Read the model definition and answer for the solid it produces. Units are mm, in the model's axes. Face numbers are marked on the shaded views. A direction names the side the tool comes from. Give positions to 0.01 mm unless a question says otherwise; leave off trailing zeros. Loops run counter-clockwise (first coordinate to the right, second up) from the corner with the lowest first, then second, coordinate; pieces in that order, holes last. Notation, with made-up numbers: (49.5, -8.5) - (54.5, -8.5) arc R23 ccw to (54.5, 9.5) - close; hole circle Ø4 at (84, -31.75). An arc over 180 degrees is marked (long way). Use a Markdown table: item, result. Add a question column.
Item 1: A cutting plane is placed at C-C (z = 6.75). Determine the outline of the cut face in (x, y).
Item 2: Consider probe 1 along Y at (x, z) = (-6, 5.25); probe 2 along Z at (x, y) = (-3, 16.5); probe 3 along Y at (x, z) = (-3, 4.5). Determine where each line is inside the solid, lowest interval first. Write a range as [from, to].
Item 3: Each of these flat-tipped pins is pushed along its axis until it touches: P1, Ø1, axis at x = 9.5, y = -0.5, coming from the -Z side; P2, Ø16, axis at x = 10.5, y = 15, coming from the +Z side; P3, Ø4, axis at x = 4, y = -8.5, coming from the +Z side; P4, Ø3, axis at x = -1, z = 7, coming from the -Y side. Where does it stop, or does it pass through?
Item 4: A cutting plane is placed at A-A (z = 3.75). Determine the outline of the cut face in (x, y).
Item 5: Which of the six approach directions +Z, -Z, +X, -X, +Y, -Y give full straight-line access (tool end or side, diameter ignored) to the marked faces 4 and 5?
Item 6: For a pull along X with two mould halves and no side action, classify the marked faces 1, 2 and 3 as +X half, -X half, draft (parallel to the pull), parting line (faces both ways), or undercut.
Item 7: A cutting plane is placed at B-B (y = 15). Determine the outline of the cut face in (x, z).
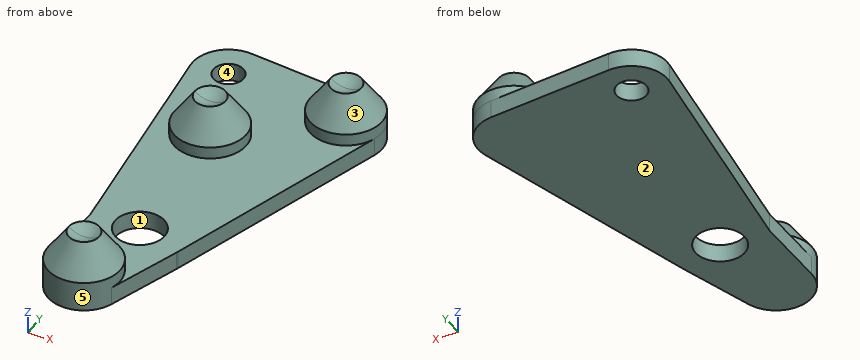
from build123d import *
from build123d.topology import SkipClean

# Parameters (mm, degrees)
BOSS_EXTRUDE1_DEPTH = 3
BOSS_EXTRUDE5_DEPTH = 3
BOSS_EXTRUDE2_DEPTH = 3
SKETCH3_R           = 4.1
CUT_EXTRUDE1_DEPTH  = 50
SKETCH1_4_R         = 6
BOSS_EXTRUDE3_DEPTH = 10
SKETCH2_4_R         = 6
BOSS_EXTRUDE4_DEPTH = 10
CHAMFER1_SIZE       = 5
CHAMFER1_SIZE_2     = 3.501037691
SKETCH9_R           = 2.5
CUT_EXTRUDE2_DEPTH  = 3


with BuildPart() as part:
    # Sketch1 → Boss-Extrude1 (new body)
    with BuildSketch(Plane.XY):
        with BuildLine():
            ThreePointArc((-7.862783113, 28.36246747), (-9.674812704, 26.016588816), (-10.142674299, 23.089524856))
            Line((-10.142674299, 23.089524856), (-7.966824047, -0.727814955))
            ThreePointArc((-7.966824047, -0.727814955), (-0.830270862, -7.956798998), (7.644946217, -2.356861757))
            Line((7.644946217, -2.356861757), (19.414515396, 35.820058514))
            ThreePointArc((19.414515396, 35.820058514), (17.084366379, 42.528936958), (9.985578884, 42.314786229))
            Line((9.985578884, 42.314786229), (-7.862783113, 28.36246747))
        make_face()
    extrude(amount=BOSS_EXTRUDE1_DEPTH)

    # Sketch8 → Boss-Extrude5 (add)
    with BuildSketch(Plane.XY):
        with BuildLine():
            Line((14.20374019, 43.56487302), (-6.42299265, 45.369478309))
            ThreePointArc((-6.42299265, 45.369478309), (-11.266837417, 43.555209842), (-12.899477398, 38.647166557))
            Line((-12.899477398, 38.647166557), (-7.938067055, -0.993524752))
            ThreePointArc((-7.938067055, -0.993524752), (-7.953555222, -0.86078995), (-7.966824047, -0.727814955))
            Line((-7.966824047, -0.727814955), (-10.142674299, 23.089524856))
            ThreePointArc((-10.142674299, 23.089524856), (-9.674812704, 26.016588816), (-7.862783113, 28.36246747))
            Line((-7.862783113, 28.36246747), (9.985578884, 42.314786229))
            ThreePointArc((9.985578884, 42.314786229), (11.97594826, 43.340396462), (14.20374019, 43.56487302))
        make_face()
    extrude(amount=BOSS_EXTRUDE5_DEPTH)

    # Sketch2 → Boss-Extrude2 (add)
    with BuildSketch(Plane.XY):
        with BuildLine():
            Line((-7.9983883, 0.16057583), (-8.256217535, -12.682068917))
            ThreePointArc((-8.256217535, -12.682068917), (-3.299315376, -18.711347307), (3.420783665, -14.741039282))
            Line((3.420783665, -14.741039282), (7.570946632, -2.584717991))
            ThreePointArc((7.570946632, -2.584717991), (-1.389185421, -7.878462024), (-7.9983883, 0.16057583))
        make_face()
    extrude(amount=BOSS_EXTRUDE2_DEPTH)

    # Sketch3 → Cut-Extrude1 (cut)
    with BuildSketch(Plane.XY.offset(3)):
        Circle(SKETCH3_R)
    extrude(amount=-CUT_EXTRUDE1_DEPTH, mode=Mode.SUBTRACT)

    # Sketch1<4> → Boss-Extrude3 (add)
    with BuildSketch(Plane.XY):
        with Locations(Location((13.680805733, 37.587704831, 0), (0, 0, 85))):
            Circle(SKETCH1_4_R)
        with Locations((-2.167556264, 25.198814555)):
            Circle(SKETCH1_4_R)
    extrude(amount=BOSS_EXTRUDE3_DEPTH)

    # Sketch2<4> → Boss-Extrude4 (add)
    with BuildSketch(Plane.XY):
        with Locations(Location((-2.25742631, -12.802500789, 0), (0, 0, 178.849883098))):
            Circle(SKETCH2_4_R)
    extrude(amount=BOSS_EXTRUDE4_DEPTH)

    # Sketch5 one side → Cut-Revolve1 (revolve, cut)
    with SkipClean():  # the faces are left unmerged after this step: merging them gives an invalid solid
        with BuildSketch(Plane(origin=(13.680805733, 0, 0), x_dir=(0, 0, -1), z_dir=(1, 0, 0))):
            with BuildLine():
                ThreePointArc((-13, 33.587704831), (-10.171572875, 34.759277707), (-9, 37.587704831))
                ThreePointArc((-9, 37.587704831), (-10.171572875, 40.416131956), (-13, 41.587704831))
                Line((-13, 41.587704831), (-13, 33.587704831))
            make_face()
        revolve(axis=Axis((13.680805733, 41.587704831, 13), (0, -1, 0)), mode=Mode.SUBTRACT)

    # Sketch6 → Cut-Revolve2 (revolve, cut)
    with SkipClean():  # the faces are left unmerged after this step: merging them gives an invalid solid
        with BuildSketch(Plane(origin=(-2.167556264, 0, 0), x_dir=(0, 0, -1), z_dir=(1, 0, 0))):
            with BuildLine():
                ThreePointArc((-9, 25.198814555), (-10.171572875, 28.02724168), (-13, 29.198814555))
                Line((-13, 29.198814555), (-13, 21.198814555))
                ThreePointArc((-13, 21.198814555), (-10.171572875, 22.37038743), (-9, 25.198814555))
            make_face()
            with BuildLine():
                Line((-13, 21.198814555), (-13, 29.198814555))
                ThreePointArc((-13, 29.198814555), (-17, 25.198814555), (-13, 21.198814555))
            make_face()
        revolve(axis=Axis((-2.167556264, 29.198814555, 13), (0, -1, 0)), mode=Mode.SUBTRACT)

    # Sketch7 → Cut-Revolve3 (revolve, cut)
    with SkipClean():  # the faces are left unmerged after this step: merging them gives an invalid solid
        with BuildSketch(Plane(origin=(-2.25742631, 0, 0), x_dir=(0, 0, -1), z_dir=(1, 0, 0))):
            with BuildLine():
                ThreePointArc((-9, -12.802500789), (-10.171572875, -9.974073664), (-13, -8.802500789))
                Line((-13, -8.802500789), (-13, -16.802500789))
                ThreePointArc((-13, -16.802500789), (-10.171572875, -15.630927914), (-9, -12.802500789))
            make_face()
            with BuildLine():
                Line((-13, -16.802500789), (-13, -8.802500789))
                ThreePointArc((-13, -8.802500789), (-17, -12.802500789), (-13, -16.802500789))
            make_face()
        revolve(axis=Axis((-2.25742631, -8.802500789, 13), (0, -1, 0)), mode=Mode.SUBTRACT)

    # Chamfer1
    # the kernel refuses this chamfer: 5, 3.501037691 mm, written as the material it takes off along each edge
    with BuildSketch(Plane(origin=(-2.25742631, -12.802500789, 10), x_dir=(-0.9997985375420249, 0.020071978697384193, 0), z_dir=(0.020071978697384193, 0.9997985375420249, 0))) as chamfer1_piece_1:
        Polygon((6, -CHAMFER1_SIZE), (6 - CHAMFER1_SIZE_2, 0), (6, 0), align=None)
    revolve(axis=Axis((-2.25742631, -12.802500789, 10), (0, 0, 1)), mode=Mode.SUBTRACT)
    with BuildSketch(Plane(origin=(13.680805733, 37.587704831, 10), x_dir=(0.08715574274765815, 0.9961946980917454, 0), z_dir=(0.9961946980917454, -0.08715574274765815, 0))) as chamfer1_piece_2:
        Polygon((6, -CHAMFER1_SIZE), (6 - CHAMFER1_SIZE_2, 0), (6, 0), align=None)
    revolve(axis=Axis((13.680805733, 37.587704831, 10), (0, 0, 1)), mode=Mode.SUBTRACT)
    with BuildSketch(Plane(origin=(-2.167556264, 25.198814555, 10), x_dir=(1, 0, 0), z_dir=(0, -1, 0))) as chamfer1_piece_3:
        Polygon((6, -CHAMFER1_SIZE), (6 - CHAMFER1_SIZE_2, 0), (6, 0), align=None)
    revolve(axis=Axis((-2.167556264, 25.198814555, 10), (0, 0, 1)), mode=Mode.SUBTRACT)

    # Sketch9 → Cut-Extrude2 (cut)
    with BuildSketch(Plane(origin=(0, 0, 0), x_dir=(-1, 0, 0), z_dir=(0, 0, -1))):
        with Locations((6.945927107, 39.39231012)):
            Circle(SKETCH9_R)
    extrude(amount=-CUT_EXTRUDE2_DEPTH, mode=Mode.SUBTRACT)


solid = part.part
Geometry says:
| question | item | result |
|---|---|---|
| 1 | outline | circle Ø9.55 at (-2.26, -12.8); circle Ø9.55 at (-2.17, 25.2); circle Ø9.55 at (13.68, 37.59) |
| 2 | probe 1 | [-17.27, -8.34], [20.81, 29.59] |
| 2 | probe 2 | [0, 3] |
| 2 | probe 3 | [-18.76, -6.85], [19.26, 31.14] |
| 3 | P1 | through |
| 3 | P2 | z = 3 |
| 3 | P3 | z = 5.58 |
| 3 | P4 | y = -18.35 |
| 4 | outline | circle Ø12 at (-2.26, -12.8); circle Ø12 at (-2.17, 25.2); circle Ø12 at (13.68, 37.59) |
| 5 | face 4 | +Z, -Z |
| 5 | face 5 | +Z |
| 6 | face 1 | undercut |
| 6 | face 2 | draft |
| 6 | face 3 | parting line |
| 7 | outline | (-9.94, 0) - (13, 0) - (13, 3) - (-9.94, 3) - close |
